from build123d import *

# Parameters (mm, degrees)
F0_W     = 762
F0_H     = 762
F0_W_2   = 334.645
F0_H_2   = 334.645
F0_W_3   = 332.105
F0_H_3   = 332.105
F1_DEPTH = 381
F2_W     = 762
F2_H     = 762
F3_DEPTH = 3.175


with BuildPart() as f1:
    # F0 (on Front) → F1 (new body)
    with BuildSketch(Plane.XZ):
        with Locations((381, -381)):
            Rectangle(F0_W, F0_H)
        with Locations((205.4225, -556.5775)):
            Rectangle(F0_W_2, F0_H_2, mode=Mode.SUBTRACT)
        with Locations((557.8475, -556.5775)):
            Rectangle(F0_W_3, F0_H_2, mode=Mode.SUBTRACT)
        with Locations((205.4225, -204.1525)):
            Rectangle(F0_W_2, F0_H_3, mode=Mode.SUBTRACT)
        with Locations((557.8475, -204.1525)):
            Rectangle(F0_W_3, F0_H_3, mode=Mode.SUBTRACT)
    extrude(amount=-F1_DEPTH)

    # F2 (on face) → F3 (join)
    with BuildSketch(Plane(origin=(0, 381, 0), x_dir=(-1, 0, 0), z_dir=(0, 1, 0))):
        with Locations((-381, -381)):
            Rectangle(F2_W, F2_H)
    extrude(amount=F3_DEPTH)


solid = f1.part
Work out the finished part from the listing and answer in its coordinate system (mm). A direction names the side the tool comes from. Give positions to 0.01 mm unless a question says otherwise; leave off trailing zeros. Order: outer loops, then holes, each group sorted by start corner. A loop starts at its lowest first (then second) coordinate and runs counter-clockwise, first axis right, second up. Notation, with made-up numbers: (3.25, 61) - (34.25, 61) arc R26 cw to (34.25, 79) - close; hole circle Ø7 at (-34.75, 60.5). An arc over 180 degrees is marked (long way). Answer as CSV lines item,"result". Start each with the question number.
Q1. Find the intervals of material crossed by L1, parallel to X at y = 161, z = -491 (3 decimals); L2, parallel to Z at x = 471, y = 204.5 (3 decimals); L3, parallel to Y at x = 558.5, z = -684 (3 decimals), in increasing order. Write a range as [from, to].
Q2. The part is cut by section C-C (x = 474). Write down the section's boundary in (y, z) (3 decimals).
Q3. Given pin 1 Ø4 at (x, z) = (246, -269.5) entering from -Y, flat-ended and moving along its own axis, determine where the tip first touches the part or whether it passes through.
Q4. For faces 4 (the face through (372.745, 188, -559)), 5 (the face through (0, 189, -386)), determine the directions among +Z, -Z, +X, -X, +Y, -Y from which every point of the face is accessible in a straight line to the end or side of a thin tool.
Q5. The mould has two halves that part along X. Classify faces 1 (the face through (386, 384.175, -376)), 2 (the face through (762, 189, -386)), 3 (the face through (38.1, 188, -559)): +X half, -X half, draft (parallel to the pull), parting line (faces both ways), or undercut.
Q6. The part is cut by section A-A (y = 143). Write down the section's boundary in (x, z) (3 decimals), then the cut area to 3 significant figures.
Q7. The part is cut by section B-B (z = -605.5). Write down the section's boundary in (x, y) (3 decimals), then the cut area to 3 significant figures.
Check result:
1,L1,"x = [0, 38.1], [372.745, 391.795], [723.9, 762]"
1,L2,"z = [-762, -723.9], [-389.255, -370.205], [-38.1, 0]"
1,L3,"y = [381, 384.175]"
2,outline,"(0, -762) - (384.175, -762) - (384.175, 0) - (0, 0) - (0, -38.1) - (381, -38.1) - (381, -370.205) - (0, -370.205) - (0, -389.255) - (381, -389.255) - (381, -723.9) - (0, -723.9) - close"
3,pin 1,"stops at y = 381"
4,face 4,"-Y"
4,face 5,"+Z, -Z, -X, +Y, -Y"
5,face 1,"draft"
5,face 2,"+X half"
5,face 3,"undercut"
6,outline,"(0, -762) - (762, -762) - (762, 0) - (0, 0) - close; hole (38.1, -723.9) - (372.745, -723.9) - (372.745, -389.255) - (38.1, -389.255) - close; hole (38.1, -370.205) - (372.745, -370.205) - (372.745, -38.1) - (38.1, -38.1) - close; hole (391.795, -723.9) - (723.9, -723.9) - (723.9, -389.255) - (391.795, -389.255) - close; hole (391.795, -370.205) - (723.9, -370.205) - (723.9, -38.1) - (391.795, -38.1) - close"
6,area,"136,000 mm²"
7,outline,"(0, 0) - (38.1, 0) - (38.1, 381) - (372.745, 381) - (372.745, 0) - (391.795, 0) - (391.795, 381) - (723.9, 381) - (723.9, 0) - (762, 0) - (762, 384.175) - (0, 384.175) - close"
7,area,"38,700 mm²"
